```python
from build123d import *

# Parameters (mm, degrees)
F0_R     = 9.525
F1_DEPTH = 127


with BuildPart() as f1:
    # F0 (on Front) → F1 (new body)
    with BuildSketch(Plane.XZ):
        with BuildLine():
            ThreePointArc((15.685102, -2.448103), (15.827454, -1.227728), (15.875, 0))
            ThreePointArc((15.875, 0), (15.827454, 1.227728), (15.685102, 2.448103))
            ThreePointArc((15.685102, 2.448103), (10.323565, 12.059835), (0, 15.875))
            ThreePointArc((0, 15.875), (-15.875, 0), (0, -15.875))
            ThreePointArc((0, -15.875), (10.323565, -12.059835), (15.685102, -2.448103))
        make_face()
        Circle(F0_R, mode=Mode.SUBTRACT)
    extrude(amount=F1_DEPTH)


solid = f1.part
```
The model under review builds one solid part; all positions refer to its coordinate system, in mm. Round coordinates to 2 decimals unless told otherwise and drop trailing zeros. Write each loop counter-clockwise with the first axis right and the second up, starting at its lowest first coordinate (ties: lowest second). Pieces come first, ordered by that corner, then holes. Notation, with made-up numbers: (-28, -28) - (-24, -28) arc R25 cw to (-24, -16) - close; hole circle Ø9 at (-9.5, 40). An arc over 180 degrees is marked (long way). One line per question, with ' | ' between items.
Item 1: To check wall thickness, follow probe 1 along X at (y, z) = (-68, -0.5); probe 2 along Z at (x, y) = (-7.5, -101.5); probe 3 along Z at (x, y) = (-8.5, -117). State the ranges of each line that lie inside material, in increasing order.
Resolved:
probe 1: x = -15.87 to -9.51, 9.51 to 15.87 | probe 2: z = -13.99 to -5.87, 5.87 to 13.99 | probe 3: z = -13.41 to -4.3, 4.3 to 13.41
Item 2: Add section A-A, the plane z = -5. Give the boundary of the cut face in (x, y).
Resolved:
outline: (-15.07, -127) - (-8.11, -127) - (-8.11, 0) - (-15.07, 0) - close; (8.11, -127) - (15.07, -127) - (15.07, 0) - (8.11, 0) - close
Item 3: For P1, Ø6, axis at y = -91, z = -8.5, coming from the -X side; P2, Ø1, axis at x = 5, y = -67, coming from the +Z side; P3, Ø1.5, axis at y = -96.5, z = -11, coming from the +X side, all flat-tipped, find the tip position at first contact; note any pin that passes through.
Resolved:
P1: stops at x = -14.89 | P2: stops at z = 15.22 | P3: stops at x = 12.12
Item 4: Add section C-C, the plane x = -12.5. Give the boundary of the cut face in (y, z), then the cut area to 3 significant figures.
Resolved:
outline: (-127, -9.79) - (0, -9.79) - (0, 9.79) - (-127, 9.79) - close | area: 2,490 mm2
Item 5: Add section B-B, the plane y = -16. Give the boundary of the cut face in (x, z) (3 decimals).
Resolved:
outline: (0, -15.875) arc R15.875 ccw to (15.685, -2.448) arc R15.875 ccw to (15.875, 0) arc R15.875 ccw to (15.685, 2.448) arc R15.875 ccw to (0, 15.875) arc R15.875 ccw to start; hole circle Ø19.05 at (0, 0)
